Can you work these out from the model? Positions are in its coordinate system, mm. A direction names the side the tool comes from. Round coordinates to 2 decimals unless told otherwise and drop trailing zeros. Loops run counter-clockwise (first coordinate to the right, second up) from the corner with the lowest first, then second, coordinate; pieces in that order, holes last.
Autodesk Inventor part; units mm, degrees
ref_plane "YZ Plane" through (0, 0, 0) normal (1, 0, 0) x (0, 1, 0)
ref_plane "XZ Plane" through (0, 0, 0) normal (0, 1, 0) x (-1, 0, 0)
ref_plane "XY Plane" through (0, 0, 0) normal (0, 0, 1) x (1, 0, 0)
sketch "Sketch1" plane through (0, 0, 0) normal (1, 0, 0) x (0, 1, 0)
  line L0 (7.148, 22.3374) -> (0.4434, 22.3374)
  line L1 (0.4434, 22.3374) -> (0.4434, 6.4624)
  line L2 (0.4434, 6.4624) -> (-5.5806, 6.4624)
  line L3 (-5.5806, 6.4624) -> (-5.5806, 2.4873)
  line L4 (-5.5806, 2.4873) -> (5.5319, 2.4873)
  line L5 (5.5319, 2.4873) -> (5.5319, 0.8998)
  line L6 (5.5319, 0.8998) -> (13.4694, 0.8998)
  line L7 (7.148, 22.3374) -> (7.1466, 26.2987)
  line L8 (7.1466, 26.2987) -> (13.468, 26.2998)
  line L9 (13.468, 26.2998) -> (13.4694, 22.3374)
  line L10 (13.4694, 22.3374) -> (13.4694, 0.8998)
  line L11 (13.4694, 0.8998) -> (-25.4371, 0.8998) construction
  line L12 (-25.4371, 0.8998) -> (-25.4371, 30.7501)
  line L13 (7.148, 22.3374) -> (13.4694, 22.3374)
  point P0 (0, 0)
  dimension "d7" = 19.05
  dimension "d8" = 7.9375
  dimension "d9" = 5.5626
  dimension "d10" = 1.5875
  dimension "d11" = 25.4
  dimension "d12" = 21.4376
  dimension "d13" = 38.9064
revolve "Revolution1" add sketch "Sketch1" angle 360 about axis through (0, -25.4371, 0.8998) along (0, 0, 1) contours L13 L10 L6 L5 L4 L3 L2 L1 L0
revolve "Revolution2" add sketch "Sketch1" angle 360 about axis through (0, -25.4371, 0.8998) along (0, 0, -1) contours L7 L8 L9 L13
sketch "Sketch3" plane through (0, -25.4371, 22.3374) normal (0, 0, 1) x (1, 0, 0)
  line L0 (0, 49.6302) -> (19.8438, 49.6302)
  line L1 (19.8438, 49.6302) -> (-19.8438, 49.6302)
  line L2 (-19.8438, 49.6302) -> (-19.8438, 12.1467)
  line L3 (-19.8438, 12.1467) -> (19.8438, 12.1467)
  line L4 (19.8438, 12.1467) -> (19.8438, 49.6302)
  point P0 (0, 25.4371)
  dimension "d18" = 19.8438
  dimension "d19" = 39.6875
extrude "Extrusion1" cut sketch "Sketch3" along normal blind 15.875
properties part number "Lower die 2 oweder ring"
(1) We'd pull the mould along Y, two halves only. Please class faces 5 (the flat face through (20, -26, 2.487)), 6 (the cylindrical face through (1.711, -64.306, 11.469)), 7 (the flat face through (19.844, 4, 24)): released by +Y, released by -Y, zero draft, split by the parting line, or undercut.
(2) For pin 1 (2 mm diameter, centred on y = -49.5, z = 20.5, fed in from -X); pin 2 (4 mm diameter, centred on x = -9, z = 22, fed in from +Y); pin 3 (4 mm diameter, centred on x = -27.5, y = -38.5, fed in from +Z), each with a flat end and sliding along its axis, tell me the tip position at first contact or that it passes through.
(3) Which directions (+Z, -Z, +X, -X, +Y, -Y) give clear straight access to the entire face, cutting with the end or side of a thin tool? Please do faces 1 (the cylindrical face through (9.302, 4.102, 1.682)), 2 (the cylindrical face through (-12.082, -41.195, 4.447)), 3 (the cylindrical face through (1.138, -51.293, 14.289)), 4 (the flat face through (-19.844, 4, 24)).
(4) Suppose I cut it at A-A (z = 17). Write out the boundary of the cut face in (x, y).
(5) If I drill on line 1 (Y direction, x = 0, z = 1.5); line 2 (X direction, y = -24.5, z = 8.75); line 3 (Y direction, x = 0, z = 3.85), over which ranges is the centre line in solid material (lowest first)?
(6) Suppose I cut it at B-B (z = 5.5). Write out the boundary of the cut face in (x, y), then the cut area to 3 significant figures.
Check result:
1. face 5: undercut
1. face 6: split by the parting line
1. face 7: zero draft
2. pin 1: stops at x = -31.33
2. pin 2: stops at y = 12.83
2. pin 3: stops at z = 22.34
3. face 1: -Z
3. face 2: +Z, -Z
3. face 3: +Z
3. face 4: +Z, +Y
4. outline: circle Ø77.81 at (0, -25.44); hole circle Ø51.76 at (0, -25.44)
5. line 1: y = -64.34 to -56.41, 5.53 to 13.47
5. line 2: x = -38.9 to -25.86, 25.86 to 38.9
5. line 3: y = -64.34 to -45.29, -5.58 to 13.47
6. outline: circle Ø77.81 at (0, -25.44); hole circle Ø39.71 at (0, -25.44)
6. area: 3,520 mm2
